Verification items for the finished model (mm, model axes). A direction names the side the tool comes from. Round coordinates to 2 decimals unless told otherwise and drop trailing zeros. Loops run counter-clockwise (first coordinate to the right, second up) from the corner with the lowest first, then second, coordinate; pieces in that order, holes last. Notation, with made-up numbers: M -27.75,70 L 20.25,70 A23 ccw 20.25,83 Z; hole C 55,82 d8. An arc over 180 degrees is marked long. Answer as CSV lines item,"result".
```python
from build123d import *

# Parameters (mm, degrees)
SKETCH1_R           = 1.75
BOSS_EXTRUDE1_DEPTH = 5


with BuildPart() as part:
    # Sketch1 → Boss-Extrude1 (new body)
    with BuildSketch(Plane(origin=(0, 0, 0), x_dir=(1, 0, 0), z_dir=(0, 1, 0))):
        with BuildLine():
            Line((6, 6), (56, 6))
            ThreePointArc((56, 6), (60.242640687, 4.242640687), (62, 0))
            Line((62, 0), (62, -4))
            ThreePointArc((62, -4), (60.242640687, -8.242640687), (56, -10))
            Line((56, -10), (6, -10))
            ThreePointArc((6, -10), (1.757359313, -8.242640687), (0, -4))
            Line((0, -4), (0, 0))
            ThreePointArc((0, 0), (1.757359313, 4.242640687), (6, 6))
        make_face()
        with Locations(Location((8, 1.25, 0), (0, 0, 270))):
            Circle(SKETCH1_R, mode=Mode.SUBTRACT)
        with Locations(Location((8, -5.25, 0), (0, 0, 90))):
            Circle(SKETCH1_R, mode=Mode.SUBTRACT)
        with BuildLine():
            Line((15.25, -7), (55.25, -7))
            ThreePointArc((55.25, -7), (57, -5.25), (55.25, -3.5))
            Line((55.25, -3.5), (15.25, -3.5))
            ThreePointArc((15.25, -3.5), (13.5, -5.25), (15.25, -7))
        make_face(mode=Mode.SUBTRACT)
        with BuildLine():
            Line((15.25, 3), (55.25, 3))
            ThreePointArc((55.25, 3), (57, 1.25), (55.25, -0.5))
            Line((55.25, -0.5), (15.25, -0.5))
            ThreePointArc((15.25, -0.5), (13.5, 1.25), (15.25, 3))
        make_face(mode=Mode.SUBTRACT)
    extrude(amount=-BOSS_EXTRUDE1_DEPTH)


solid = part.part
```
1) Section check A-A (y = -3.35). Record the cut outline in (x, z), plus the area to 3 significant figures.
Here are the results:
outline,"M 0,0 A6 ccw 6,-6 L 56,-6 A6 ccw 62,0 L 62,4 A6 ccw 56,10 L 6,10 A6 ccw 0,4 Z; hole C 8,-1.25 d3.5; hole C 8,5.25 d3.5; hole M 15.25,-3 L 55.25,-3 A1.75 ccw 55.25,0.5 L 15.25,0.5 A1.75 ccw Z; hole M 15.25,3.5 L 55.25,3.5 A1.75 ccw 55.25,7 L 15.25,7 A1.75 ccw Z"
area,"643 mm^2"
2) Draft check along X on faces 3 (the flat face through (35, -2, 7)), 4 (the cylindrical face through (60.289, -2.465, 8.196)), 5 (the cylindrical face through (1.804, -2.465, 8.289)), 6 (the flat face through (36, -2, 3.5)). Enter one of: +X half, -X half, draft (parallel to the pull), parting line (faces both ways), or undercut.
Here are the results:
face 3,"undercut"
face 4,"+X half"
face 5,"-X half"
face 6,"undercut"
3) Section check B-B (x = 8). Record the cut outline in (y, z).
Here are the results:
outline,"M -5,-6 L 0,-6 L 0,-3 L -5,-3 Z; M -5,0.5 L 0,0.5 L 0,3.5 L -5,3.5 Z; M -5,7 L 0,7 L 0,10 L -5,10 Z"
4) Go/stop test with a flat-tipped pin: pin 1 (2 mm diameter, centred on y = -1.5, z = 6.5, fed in from +X). Record where the tip stops, or that it passes through.
Here are the results:
pin 1,"stops at x = 61.81"
5) Material ranges on probe 1 along Z at (x, y) = (37, -0.85); probe 2 along X at (y, z) = (-1.1, -1.25); probe 3 along X at (y, z) = (-2.25, 4), recorded low to high.
Here are the results:
probe 1,"z = -6 to -3, 0.5 to 3.5, 7 to 10"
probe 2,"x = 0.13 to 6.25, 9.75 to 13.5, 57 to 61.87"
probe 3,"x = 0 to 6.78, 9.22 to 14.03, 56.47 to 62"
6) Section check C-C (z = 5.25). Record the cut outline in (x, y), plus the area to 3 significant figures.
Here are the results:
outline,"M 0.13,-5 L 6.25,-5 L 6.25,0 L 0.13,0 Z; M 9.75,-5 L 13.5,-5 L 13.5,0 L 9.75,0 Z; M 57,-5 L 61.87,-5 L 61.87,0 L 57,0 Z"
area,"73.7 mm^2"
7) Section check D-D (z = 9). Record the cut outline in (x, y), plus the area to 3 significant figures.
Here are the results:
outline,"M 2.68,-5 L 59.32,-5 L 59.32,0 L 2.68,0 Z"
area,"283 mm^2"
8) Set-up check for faces 1 (the cylindrical face through (57, -2.5, -1.3)), 2 (the cylindrical face through (1.711, -2.465, -4.196)): record each of +Z, -Z, +X, -X, +Y, -Y from which the full face is reachable in a straight line by a thin tool's end or side.
Here are the results:
face 1,"+Y, -Y"
face 2,"-Z, -X, +Y, -Y"
